```python
from build123d import *

# Parameters (mm, degrees)
F1_DEPTH  = 4.7625
F2_W      = 23.6109700747
F2_H      = 10.16
F2_W_2    = 21.1328
F3_DEPTH  = 25.4
F4_R      = 2.5
F5_DEPTH  = 25.4
F6_R      = 1.3330740387
F7_DEPTH  = 25.4
F2_R      = 2.0828
F8_DEPTH  = 25.4
F10_DEPTH = 25.4


# Not quite as in the source:
# - a feature names something its author has since deleted; it is built from what else it names


with BuildPart() as f1:
    # F0 (on Top) → F1 (new body)
    with BuildSketch(Plane.XY):
        Polygon((45.72, 53.975), (33.02, 53.975), (-33.02, 53.975), (-33.02, -53.975), (33.02, -53.975), (33.02, -12.7), (45.72, -12.7), align=None)
    extrude(amount=F1_DEPTH)

    # F2 (on face) → F3 (cut)
    with BuildSketch(Plane.XY.offset(4.7625)):
        with Locations((-5.4554850374, 36.7538)):
            Rectangle(F2_W, F2_H)
        with Locations((16.9164, 36.7538)):
            Rectangle(F2_W_2, F2_H)
        with BuildLine():
            ThreePointArc((29.5656, 23.241), (28.9555620039, 24.7137620039), (27.4828, 25.3238))
            Line((27.4828, 25.3238), (27.4828, 21.1582))
            ThreePointArc((27.4828, 21.1582), (28.9555620039, 21.7682379961), (29.5656, 23.241))
        make_face()
        with BuildLine():
            Line((27.4828, 21.1582), (27.4828, 25.3238))
            ThreePointArc((27.4828, 25.3238), (25.4, 23.241), (27.4828, 21.1582))
        make_face()
        with BuildLine():
            ThreePointArc((27.4828, -0.8382), (25.4, -2.921), (27.4828, -5.0038))
            Line((27.4828, -5.0038), (27.4828, -0.8382))
        make_face()
        with BuildLine():
            Line((27.4828, -0.8382), (27.4828, -5.0038))
            ThreePointArc((27.4828, -5.0038), (28.9555620039, -4.3937620039), (29.5656, -2.921))
            ThreePointArc((29.5656, -2.921), (28.9555620039, -1.4482379961), (27.4828, -0.8382))
        make_face()
        with BuildLine():
            ThreePointArc((-15.24, 23.241), (-15.8500379961, 24.7137620039), (-17.3228, 25.3238))
            Line((-17.3228, 25.3238), (-17.3228, 21.1582))
            ThreePointArc((-17.3228, 21.1582), (-15.8500379961, 21.7682379961), (-15.24, 23.241))
        make_face()
        with BuildLine():
            Line((-17.3228, 21.1582), (-17.3228, 25.3238))
            ThreePointArc((-17.3228, 25.3238), (-19.4056, 23.241), (-17.3228, 21.1582))
        make_face()
        with BuildLine():
            ThreePointArc((-17.3228, -0.8382), (-19.4056, -2.921), (-17.3228, -5.0038))
            Line((-17.3228, -5.0038), (-17.3228, -0.8382))
        make_face()
        with BuildLine():
            Line((-17.3228, -0.8382), (-17.3228, -5.0038))
            ThreePointArc((-17.3228, -5.0038), (-15.8500379961, -4.3937620039), (-15.24, -2.921))
            ThreePointArc((-15.24, -2.921), (-15.8500379961, -1.4482379961), (-17.3228, -0.8382))
        make_face()
    extrude(amount=-F3_DEPTH, mode=Mode.SUBTRACT)

    # F4 (on face) → F5 (cut)
    with BuildSketch(Plane(origin=(0, 0, 0), x_dir=(1, 0, 0), z_dir=(0, 0, -1))):
        with Locations((0, 5.08)):
            Circle(F4_R)
    extrude(amount=-F5_DEPTH, mode=Mode.SUBTRACT)

    # F6 (on face) → F7 (cut)
    with BuildSketch(Plane.XY.offset(4.7625)):
        with BuildLine():
            Line((0, -28.178125), (0, -25.796875))
            ThreePointArc((0, -25.796875), (-1.190625, -26.9875), (0, -28.178125))
        make_face()
        with BuildLine():
            ThreePointArc((0, -28.178125), (0.8418990114, -27.8293990114), (1.190625, -26.9875))
            ThreePointArc((1.190625, -26.9875), (0.8418990114, -26.1456009886), (0, -25.796875))
            Line((0, -25.796875), (0, -28.178125))
        make_face()
        with Locations((29.460657388, -26.9875)):
            Circle(F6_R)
    extrude(amount=-F7_DEPTH, mode=Mode.SUBTRACT)

    # F2 (on face) → F8 (cut)
    with BuildSketch(Plane.XY.offset(4.7625)):
        with Locations((-20.9680330008, 49.9618)):
            Circle(F2_R)
        with BuildLine():
            ThreePointArc((23.6728, 49.9618), (21.59, 52.0446), (19.5072, 49.9618))
            ThreePointArc((19.5072, 49.9618), (21.59, 47.879), (23.6728, 49.9618))
        make_face()
    extrude(amount=-F8_DEPTH, mode=Mode.SUBTRACT)

    # F9 (on face) → F10 (cut)
    with BuildSketch(Plane.XY.offset(4.7625)):
        with BuildLine():
            Line((-29.464, -48.5479413316), (-29.464, -52.1039413316))
            ThreePointArc((-29.464, -52.1039413316), (-28.2067641431, -51.5831771885), (-27.686, -50.3259413316))
            ThreePointArc((-27.686, -50.3259413316), (-28.2067641431, -49.0687054746), (-29.464, -48.5479413316))
        make_face()
        with BuildLine():
            ThreePointArc((-29.464, -48.5479413316), (-31.242, -50.3259413316), (-29.464, -52.1039413316))
            Line((-29.464, -52.1039413316), (-29.464, -48.5479413316))
        make_face()
        with BuildLine():
            ThreePointArc((-27.686, -42.0469199679), (-28.2067641431, -40.7896841109), (-29.464, -40.2689199679))
            Line((-29.464, -40.2689199679), (-29.464, -43.8249199679))
            ThreePointArc((-29.464, -43.8249199679), (-28.2067641431, -43.3041558248), (-27.686, -42.0469199679))
        make_face()
        with BuildLine():
            Line((-29.464, -43.8249199679), (-29.464, -40.2689199679))
            ThreePointArc((-29.464, -40.2689199679), (-31.242, -42.0469199679), (-29.464, -43.8249199679))
        make_face()
        with BuildLine():
            Line((-3.302, -43.8249199679), (-3.302, -40.2689199679))
            ThreePointArc((-3.302, -40.2689199679), (-5.08, -42.0469199679), (-3.302, -43.8249199679))
        make_face()
        with BuildLine():
            ThreePointArc((-1.524, -42.0469199679), (-2.0447641431, -40.7896841109), (-3.302, -40.2689199679))
            Line((-3.302, -40.2689199679), (-3.302, -43.8249199679))
            ThreePointArc((-3.302, -43.8249199679), (-2.0447641431, -43.3041558248), (-1.524, -42.0469199679))
        make_face()
        with BuildLine():
            ThreePointArc((-3.302, -48.5479413316), (-5.08, -50.3259413316), (-3.302, -52.1039413316))
            Line((-3.302, -52.1039413316), (-3.302, -48.5479413316))
        make_face()
        with BuildLine():
            Line((-3.302, -48.5479413316), (-3.302, -52.1039413316))
            ThreePointArc((-3.302, -52.1039413316), (-2.0447641431, -51.5831771885), (-1.524, -50.3259413316))
            ThreePointArc((-1.524, -50.3259413316), (-2.0447641431, -49.0687054746), (-3.302, -48.5479413316))
        make_face()
        with BuildLine():
            ThreePointArc((3.302, -48.5479413316), (1.524, -50.3259413316), (3.302, -52.1039413316))
            Line((3.302, -52.1039413316), (3.302, -48.5479413316))
        make_face()
        with BuildLine():
            Line((3.302, -48.5479413316), (3.302, -52.1039413316))
            ThreePointArc((3.302, -52.1039413316), (4.5592358569, -51.5831771885), (5.08, -50.3259413316))
            ThreePointArc((5.08, -50.3259413316), (4.5592358569, -49.0687054746), (3.302, -48.5479413316))
        make_face()
        with BuildLine():
            ThreePointArc((5.08, -42.0469199679), (4.5592358569, -40.7896841109), (3.302, -40.2689199679))
            Line((3.302, -40.2689199679), (3.302, -43.8249199679))
            ThreePointArc((3.302, -43.8249199679), (4.5592358569, -43.3041558248), (5.08, -42.0469199679))
        make_face()
        with BuildLine():
            Line((3.302, -43.8249199679), (3.302, -40.2689199679))
            ThreePointArc((3.302, -40.2689199679), (1.524, -42.0469199679), (3.302, -43.8249199679))
        make_face()
        with BuildLine():
            Line((29.464, -43.8249199679), (29.464, -40.2689199679))
            ThreePointArc((29.464, -40.2689199679), (27.686, -42.0469199679), (29.464, -43.8249199679))
        make_face()
        with BuildLine():
            ThreePointArc((31.242, -42.0469199679), (30.7212358569, -40.7896841109), (29.464, -40.2689199679))
            Line((29.464, -40.2689199679), (29.464, -43.8249199679))
            ThreePointArc((29.464, -43.8249199679), (30.7212358569, -43.3041558248), (31.242, -42.0469199679))
        make_face()
        with BuildLine():
            Line((29.464, -48.5479413316), (29.464, -52.1039413316))
            ThreePointArc((29.464, -52.1039413316), (30.7212358569, -51.5831771885), (31.242, -50.3259413316))
            ThreePointArc((31.242, -50.3259413316), (30.7212358569, -49.0687054746), (29.464, -48.5479413316))
        make_face()
        with BuildLine():
            ThreePointArc((29.464, -48.5479413316), (27.686, -50.3259413316), (29.464, -52.1039413316))
            Line((29.464, -52.1039413316), (29.464, -48.5479413316))
        make_face()
    extrude(amount=-F10_DEPTH, mode=Mode.SUBTRACT)


solid = f1.part
```
Here's how the part is built. I have some questions about the finished solid (model axes, mm). A direction names the side the tool comes from. Coordinates: 2 decimals unless noted, no trailing zeros. Order: outer loops, then holes, each group sorted by start corner. A loop starts at its lowest first (then second) coordinate and runs counter-clockwise, first axis right, second up. Notation, with made-up numbers: M 19.5,7 L 52.5,7 A28 ccw 52.5,27 Z; hole C -28,27 d6. An arc over 180 degrees is marked long. Answer as a JSON object with one key per item and string values. Group by question number.
(1) Suppose I cut it at B-B, the plane x = -14. Please give me the cut outline in (y, z) (1 decimal).
(2) Which directions (+Z, -Z, +X, -X, +Y, -Y) give clear straight access to the entire face, cutting with the end or side of a thin tool? Please do faces 5 (the face through (6, 1, 0)), 6 (the face through (-17.261, 37, 2)), 7 (the face through (33.02, -34, 2)).
(3) I need wall thicknesses on probe 1 along Y at (x, z) = (-15, 0.75) (3 decimals); probe 2 along X at (y, z) = (40, 2.9); probe 3 along X at (y, z) = (-17, 3.75). Which ranges of each line are inside material? Lowest first, please.
(4) If we mould it in two halves opening along Y, with no side actions, what happens to faces 1 (the face through (45.72, 20, 2)), 2 (the face through (39, -12.7, 2)), 3 (the face through (-0.54, -2.64, 2.35)), 4 (the face through (5, 41.834, 2))? For each: released by +Y, released by -Y, zero draft, split by the parting line, or undercut.
(5) Suppose I cut it at A-A, the plane x = 21.59. Please give me the cut outline in (y, z) (1 decimal).
(6) Suppose I cut it at C-C, the plane x = 39. Please give me the cut outline in (y, z) (1 decimal), then the cut area to 3 significant figures.
(7) Suppose I cut it at D-D, the plane z = 2.15. State how many separate pieces and enclosed holes the cut face has, then the cut area to 3 significant figures.
(8) For pin 1 (2.5 mm diameter, centred on x = 38, z = 1.5, fed in from -Y); pin 2 (1.5 mm diameter, centred on y = -24, z = 4, fed in from +X), each with a flat end and sliding along its axis, tell me the tip position at first contact or that it passes through.
Values found:
{
 "1": {"outline": "M -54,0 L 31.7,0 L 31.7,4.8 L -54,4.8 Z; M 41.8,0 L 54,0 L 54,4.8 L 41.8,4.8 Z"},
 "2": {"face 5": "-Z, +X, -X, +Y, -Y", "face 6": "+Z, -Z", "face 7": "+Z, -Z, +X, -Y"},
 "3": {"probe 1": "y = -53.975 to 31.674, 41.834 to 53.975", "probe 2": "x = -33.02 to -17.26, 27.48 to 45.72", "probe 3": "x = -33.02 to 33.02"},
 "4": {"face 1": "zero draft", "face 2": "released by -Y", "face 3": "undercut", "face 4": "undercut"},
 "5": {"outline": "M -54,0 L 31.7,0 L 31.7,4.8 L -54,4.8 Z; M 41.8,0 L 47.9,0 L 47.9,4.8 L 41.8,4.8 Z; M 52,0 L 54,0 L 54,4.8 L 52,4.8 Z"},
 "6": {"outline": "M -12.7,0 L 54,0 L 54,4.8 L -12.7,4.8 Z", "area": "318 mm^2"},
 "7": {"separate pieces": "1", "enclosed holes": "18", "area": "7,330 mm^2"},
 "8": {"pin 1": "stops at y = -12.7", "pin 2": "stops at x = 33.02"}
}
